```python
from build123d import *

# Parameters (mm, degrees)
SKETCH1_R           = 4
SKETCH1_R_2         = 2.6
BOSS_EXTRUDE1_DEPTH = 4.4
SKETCH2_R           = 0.5
SKETCH2_R_2         = 1
BOSS_EXTRUDE2_DEPTH = 1.6
SKETCH3_R           = 3.5
BOSS_EXTRUDE3_DEPTH = 0.8
SKETCH4_R           = 2.9
CUT_EXTRUDE1_DEPTH  = 1.3
FILLET1_R           = 0.1
CUT_EXTRUDE2_DEPTH  = 2.8
CIRPATTERN1_COUNT   = 23


with BuildPart() as part:
    # Sketch1 → Boss-Extrude1 (new body)
    with BuildSketch(Plane(origin=(0, 0, 0), x_dir=(1, 0, 0), z_dir=(0, 1, 0))):
        with Locations(Location((0, 0, 0), (0, 0, 270))):
            Circle(SKETCH1_R)
        with Locations(Location((0, 0, 0), (0, 0, 270))):
            Circle(SKETCH1_R_2, mode=Mode.SUBTRACT)
    extrude(amount=BOSS_EXTRUDE1_DEPTH)

    # Sketch2 → Boss-Extrude2 (add)
    with BuildSketch(Plane(origin=(0, 4.4, 0), x_dir=(1, 0, 0), z_dir=(0, 1, 0))):
        with BuildLine():
            Line((0, 2.9), (12.642815505, 1.994894416))
            ThreePointArc((12.642815505, 1.994894416), (14.5, 0), (12.642815505, -1.994894416))
            Line((12.642815505, -1.994894416), (0, -2.9))
            Line((0, -2.9), (-12.642815505, -1.994894416))
            ThreePointArc((-12.642815505, -1.994894416), (-14.5, 0), (-12.642815505, 1.994894416))
            Line((-12.642815505, 1.994894416), (0, 2.9))
        make_face()
        with Locations(Location((12.5, 0, 0), (0, 0, 270))):
            Circle(SKETCH2_R, mode=Mode.SUBTRACT)
        with Locations(Location((10, 0, 0), (0, 0, 270))):
            Circle(SKETCH2_R, mode=Mode.SUBTRACT)
        with Locations(Location((7.5, 0, 0), (0, 0, 270))):
            Circle(SKETCH2_R, mode=Mode.SUBTRACT)
        with Locations(Location((-7.5, 0, 0), (0, 0, 270))):
            Circle(SKETCH2_R, mode=Mode.SUBTRACT)
        with Locations(Location((-10, 0, 0), (0, 0, 270))):
            Circle(SKETCH2_R, mode=Mode.SUBTRACT)
        with Locations(Location((-12.5, 0, 0), (0, 0, 270))):
            Circle(SKETCH2_R, mode=Mode.SUBTRACT)
        with Locations(Location((0, 0, 0), (0, 0, 270))):
            Circle(SKETCH2_R_2, mode=Mode.SUBTRACT)
    extrude(amount=-BOSS_EXTRUDE2_DEPTH)

    # Sketch3 → Boss-Extrude3 (add)
    with BuildSketch(Plane(origin=(0, 4.4, 0), x_dir=(-1, 0, 0), z_dir=(0, -1, 0))):
        with Locations(Location((0, 0, 0), (0, 0, 90))):
            Circle(SKETCH3_R)
    extrude(amount=-BOSS_EXTRUDE3_DEPTH)

    # Sketch4 → Cut-Extrude1 (cut)
    with BuildSketch(Plane(origin=(0, 5.2, 0), x_dir=(1, 0, 0), z_dir=(0, 1, 0))):
        with Locations(Location((0, 0, 0), (0, 0, 270))):
            Circle(SKETCH4_R)
    extrude(amount=-CUT_EXTRUDE1_DEPTH, mode=Mode.SUBTRACT)

    # Fillet1
    fillet1_edges = [part.edges().sort_by_distance(p)[0] for p in [
        (0, 5.2, 3.5),
    ]]
    fillet(fillet1_edges, radius=FILLET1_R)

    # Sketch5 → Cut-Extrude2 (cut)
    with BuildSketch(Plane.XZ):
        Polygon((-0.466249863, 2.460177118), (0.466249863, 2.460177118), (0, 2.926426981), align=None)
    cut_extrude2 = extrude(amount=-CUT_EXTRUDE2_DEPTH, mode=Mode.SUBTRACT)

    # CirPattern1: Cut-Extrude2 ×23 about axis
    cirpattern1_axis = Axis((0, 0, 0), (0, 1, 0))
    for i in range(1, CIRPATTERN1_COUNT):
        add(cut_extrude2.rotate(cirpattern1_axis, i * 360 / CIRPATTERN1_COUNT), mode=Mode.SUBTRACT)


solid = part.part
```
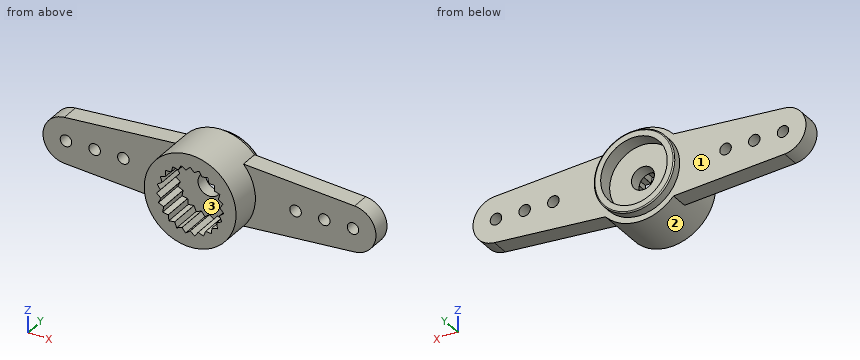
Part model, mm, in its own coordinate system. Face numbers are marked on the shaded views. Give positions to 0.01 mm unless a question says otherwise; leave off trailing zeros. Order: outer loops, then holes, each group sorted by start corner. A loop starts at its lowest first (then second) coordinate and runs counter-clockwise, first axis right, second up. Notation, with made-up numbers: M 31,60 L 54,60 A29 ccw 54,92 Z; hole C 67.25,54.5 d4. An arc over 180 degrees is marked long. Use a Markdown table: item, result. Add a question column.
(1) Saw through at D-D, the plane x = -11.5. Give the cut face in (y, z), and give its area (3 significant figures).
(2) Saw through at B-B, the plane x = -7.5. Give the cut face in (y, z).
(3) Probe line 1 along X through (y, z) = (4.85, -2.5); line 2 along Z through (x, y) = (-0.5, 0.25); line 3 along Y through (x, z) = (5.5, 1). List the from-to ranges inside material, lowest first. Write a range as [from, to].
(4) Saw through at C-C, the plane y = 4.65. Give the cut face in (x, z).
(5) Mould opens along X. For the marked faces 1, 2 and 3 say: +X half, -X half, draft (parallel to the pull), parting line (faces both ways), or undercut.
(6) Saw through at A-A, the plane y = 3.4. Give the cut face in (x, z).
(7) Drop flat-ended pins along their axis: P1, Ø1.7, axis at x = -0.5, z = -1, coming from the +Y side; P2, Ø2, axis at x = 7, z = -1.5, coming from the +Y side; P3, Ø1.6, axis at x = 11, z = 1, coming from the -Y side. Give the stop position or say it passes through.
Answer key:
| question | item | result |
|---|---|---|
| 1 | outline | M 2.8,-2.08 L 4.4,-2.08 L 4.4,2.08 L 2.8,2.08 Z |
| 1 | area | 6.65 mm^2 |
| 2 | outline | M 2.8,-2.36 L 4.4,-2.36 L 4.4,-0.5 L 2.8,-0.5 Z; M 2.8,0.5 L 4.4,0.5 L 4.4,2.36 L 2.8,2.36 Z |
| 3 | line 1 | [-2.45, -1.47], [1.47, 2.45] |
| 3 | line 2 | [-3.97, -2.77], [2.66, 3.97] |
| 3 | line 3 | [2.8, 4.4] |
| 4 | outline | C 0,0 d7; hole C 0,0 d5.8 |
| 5 | face 1 | draft |
| 5 | face 2 | parting line |
| 5 | face 3 | undercut |
| 6 | outline | M -12.64,-1.99 L -2.96,-2.69 A4 ccw 2.96,-2.69 L 12.64,-1.99 A2 ccw 12.64,1.99 L 2.96,2.69 A4 ccw -2.96,2.69 L -12.64,1.99 A2 ccw Z; hole C -12.5,0 d1; hole C -10,0 d1; hole C -7.5,0 d1; hole C 0,0 d2; hole C 7.5,0 d1; hole C 10,0 d1; hole C 12.5,0 d1 |
| 7 | P1 | y = 3.9 |
| 7 | P2 | y = 4.4 |
| 7 | P3 | y = 2.8 |
